from build123d import *

# Parameters (mm, degrees)
CROQUIS1_W                    = 380
CROQUIS1_H                    = 3.175
BRIDA_BASE1_DEPTH             = 25.4
BRIDA_DE_ARISTA1_DEPTH        = 25.4
BRIDA_DE_ARISTA1_BEND_DEPTH   = 25.4
BRIDA_DE_ARISTA2_DEPTH        = 25.4
BRIDA_DE_ARISTA2_BEND_DEPTH   = 25.4
TALADRO_DE_MARGEN_PARA_3_81_D = 10.0838


# Sheet-metal steps are written as plain solids
with BuildPart() as part:
    # Croquis1 → Brida base1 (new body)
    with BuildSketch(Plane.XY):
        with Locations((113.920112782, -1.5875)):
            Rectangle(CROQUIS1_W, CROQUIS1_H)
    extrude(amount=BRIDA_BASE1_DEPTH)

    # Brida de arista1 section (across the edge) → Brida de arista1 (add)
    with BuildSketch(Plane(origin=(304.656712782, -3.175, 0), x_dir=(-1, 0, 0), z_dir=(0, 0, 1))):
        with BuildLine():
            Line((-3.175, 0.7366), (-3.175, 256.825))
            Line((-3.175, 256.825), (0, 256.825))
            Line((0, 256.825), (0, 0.7366))
            ThreePointArc((0, 0.7366), (0.215745145, 0.215745145), (0.7366, 0))
            Line((0.7366, 0), (0.7366, -3.175))
            ThreePointArc((0.7366, -3.175), (-2.029318885, -2.029318885), (-3.175, 0.7366))
        make_face()
    extrude(amount=BRIDA_DE_ARISTA1_DEPTH)

    # Brida de arista1 section 2 (across the edge) → Brida de arista1 bend (add)
    with BuildSketch(Plane(origin=(-76.816487218, -3.175, 25.4), x_dir=(1, 0, 0), z_dir=(0, 0, -1))):
        with BuildLine():
            Line((-3.175, 0.7366), (-3.175, 256.825))
            Line((-3.175, 256.825), (0, 256.825))
            Line((0, 256.825), (0, 0.7366))
            ThreePointArc((0, 0.7366), (0.215745145, 0.215745145), (0.7366, 0))
            Line((0.7366, 0), (0.7366, -3.175))
            ThreePointArc((0.7366, -3.175), (-2.029318885, -2.029318885), (-3.175, 0.7366))
        make_face()
    extrude(amount=BRIDA_DE_ARISTA1_BEND_DEPTH)

    # Brida de arista2 section (across the edge) → Brida de arista2 (add)
    with BuildSketch(Plane(origin=(307.831712782, -260.7366, 25.4), x_dir=(0, 1, 0), z_dir=(0, 0, -1))):
        with BuildLine():
            Line((-3.175, 0.7366), (-3.175, 24.825))
            Line((-3.175, 24.825), (0, 24.825))
            Line((0, 24.825), (0, 0.7366))
            ThreePointArc((0, 0.7366), (0.215745145, 0.215745145), (0.7366, 0))
            Line((0.7366, 0), (0.7366, -3.175))
            ThreePointArc((0.7366, -3.175), (-2.029318885, -2.029318885), (-3.175, 0.7366))
        make_face()
    extrude(amount=BRIDA_DE_ARISTA2_DEPTH)

    # Brida de arista2 section 2 (across the edge) → Brida de arista2 bend (add)
    with BuildSketch(Plane(origin=(-79.991487218, -260.7366, 0), x_dir=(0, 1, 0), z_dir=(0, 0, 1))):
        with BuildLine():
            Line((-3.175, 0.7366), (-3.175, 24.825))
            Line((-3.175, 24.825), (0, 24.825))
            Line((0, 24.825), (0, 0.7366))
            ThreePointArc((0, 0.7366), (0.215745145, 0.215745145), (0.7366, 0))
            Line((0.7366, 0), (0.7366, -3.175))
            ThreePointArc((0.7366, -3.175), (-2.029318885, -2.029318885), (-3.175, 0.7366))
        make_face()
    extrude(amount=BRIDA_DE_ARISTA2_BEND_DEPTH)

    # Taladro de margen para 3/81 (through all)
    with Locations(Plane(origin=(0, -263.9116, 0), x_dir=(-1, 0, 0), z_dir=(0, -1, 0))):
        with Locations((92.816487218, -12.7), (-320.656712782, -12.7)):
            Hole(TALADRO_DE_MARGEN_PARA_3_81_D / 2)


solid = part.part
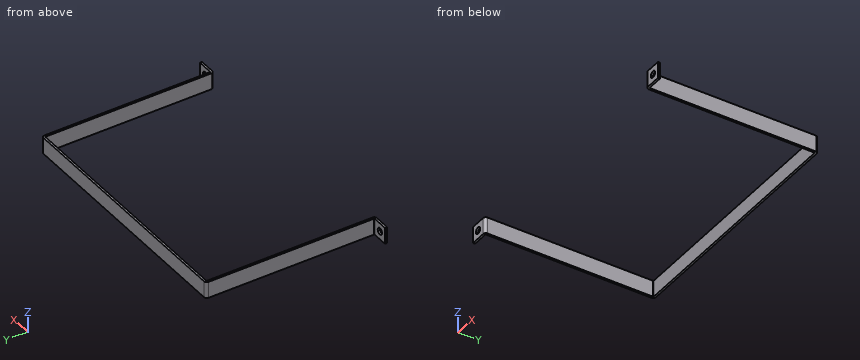
Can you work these out from the model? Positions are in its coordinate system, mm. Give positions to 0.01 mm unless a question says otherwise; leave off trailing zeros. Write each loop counter-clockwise with the first axis right and the second up, starting at its lowest first coordinate (ties: lowest second). Pieces come first, ordered by that corner, then holes. Notation, with made-up numbers: (11, 0) -> (20, 0) arc R19 cw to (20, 13) -> close; hole circle Ø3 at (77, 60.5). An arc over 180 degrees is marked (long way). Answer as a JSON object with one key per item and string values. Group by question number.
Item 1: Suppose I cut it at B-B (z = 12.7). Please give me the cut outline in (x, y) (3 decimals).
Item 2: Suppose I cut it at C-C (x = 97.5). Please give me the cut outline in (y, z) (3 decimals), plus the area to 3 significant figures.
Item 3: Suppose I cut it at A-A (y = -218). Please give me the cut outline in (x, z), plus the area to 3 significant figures.
Item 4: I'm going to push flat-ended pins straight in: P1, Ø7.5, axis at x = 64.5, z = 15.5, coming from the -Y side (3 decimals); P2, Ø5, axis at y = -223.5, z = 20.5, coming from the +X side; P3, Ø7.5, axis at y = -176.5, z = 8.5, coming from the -X side. Where does each tip first touch, or does it pass through?
Item 5: Please list where these lines run through material, in increasing order: line 1 (X direction, y = -158, z = 8); line 2 (Y direction, x = 2, z = 24.75) (3 decimals); line 3 (Y direction, x = -86.5, z = 11.5). Write a range as [from, to].
Findings:
{
 "1": {"outline": "(-104.816, -263.912) -> (-97.858, -263.912) -> (-97.858, -260.737) -> (-104.816, -260.737) -> close; (-87.775, -263.912) -> (-80.728, -263.912) arc R3.912 ccw to (-76.816, -260) -> (-76.816, -3.912) arc R0.737 cw to (-76.08, -3.175) -> (303.92, -3.175) arc R0.737 cw to (304.657, -3.912) -> (304.657, -260) arc R3.912 ccw to (308.568, -263.912) -> (315.615, -263.912) -> (315.615, -260.737) -> (308.568, -260.737) arc R0.737 cw to (307.832, -260) -> (307.832, -3.912) arc R3.912 ccw to (303.92, 0) -> (-76.08, 0) arc R3.912 ccw to (-79.991, -3.912) -> (-79.991, -260) arc R0.737 cw to (-80.728, -260.737) -> (-87.775, -260.737) -> close; (325.699, -263.912) -> (332.657, -263.912) -> (332.657, -260.737) -> (325.699, -260.737) -> close"},
 "2": {"outline": "(-3.175, 0) -> (0, 0) -> (0, 25.4) -> (-3.175, 25.4) -> close", "area": "80.6 mm²"},
 "3": {"outline": "(-79.99, 0) -> (-76.82, 0) -> (-76.82, 25.4) -> (-79.99, 25.4) -> close; (304.66, 0) -> (307.83, 0) -> (307.83, 25.4) -> (304.66, 25.4) -> close", "area": "161 mm²"},
 "4": {"P1": "stops at y = -3.175", "P2": "stops at x = 307.83", "P3": "stops at x = -79.99"},
 "5": {"line 1": "x = [-79.99, -76.82], [304.66, 307.83]", "line 2": "y = [-3.175, 0]", "line 3": "y = [-263.91, -260.74]"}
}
